Autodesk Inventor part; units mm, degrees
ref_plane "YZ Plane" through (0, 0, 0) normal (1, 0, 0) x (0, 1, 0)
ref_plane "XZ Plane" through (0, 0, 0) normal (0, 1, 0) x (-1, 0, 0)
ref_plane "XY Plane" through (0, 0, 0) normal (0, 0, 1) x (1, 0, 0)
sketch "Sketch1" plane through (0, 0, 0) normal (0, 0, 1) x (1, 0, 0)
  line L0 (0, 0) -> (12, 0)
  line L1 (12, 0) -> (12, 10.5)
  line L2 (12, 10.5) -> (0, 10.5)
  line L3 (0, 10.5) -> (0, 0)
  dimension "d0" = 12
  dimension "d2" = 10.5
extrude "Extrusion1" add sketch "Sketch1" along normal blind 16
fillet "Fillet1" radius 2 4 edges at (12, 10.5, 8) (0, 10.5, 8) (12, 0, 8) (0, 0, 8)
sketch "Sketch2" plane through (0, 0, 16) normal (0, 0, 1) x (1, 0, 0)
  line L0 (12, 2) -> (12, 8.5)
  line L1 (10, 10.5) -> (2, 10.5)
  line L2 (0, 8.5) -> (0, 2)
  line L3 (2, 0) -> (10, 0)
  arc A0 (12, 8.5) -> (10, 10.5) centre (10, 8.5) ccw
  line L4 (12, 8.5) -> (12, 10.5)
  line L5 (12, 10.5) -> (10, 10.5)
  line L6 (2, 10.5) -> (0, 10.5)
  line L7 (0, 10.5) -> (0, 8.5)
  arc A1 (0, 2) -> (2, 0) centre (2, 2) ccw
  line L8 (2, 0) -> (0, 0)
  line L9 (0, 0) -> (2, 0)
  line L10 (12, 2) -> (12, 0)
  arc A2 (10, 0) -> (12, 2) centre (10, 2) ccw
  line L11 (12, 0) -> (10, 0)
  line L12 (0, 0) -> (0, 2)
extrude "Extrusion2" add sketch "Sketch2" along normal blind 9
sketch "Sketch3" plane through (0, 0, 25) normal (0, 0, 1) x (1, 0, 0)
  line L0 (10, 10.5) -> (2, 10.5)
  line L1 (6, 10.5) -> (6, 0)
  line L2 (2, 0) -> (10, 0)
  circle A0 centre (6, 5.25) radius 1.5
  point P0 (0, 0)
  dimension "d8" = 3
extrude "Extrusion3" add sketch "Sketch3" along normal blind 8.5
properties part number "MicroMotor"
Input: part model. Units: mm. Frame: model coordinates. A direction names the side the tool comes from. Coordinates: 2 decimals unless noted, no trailing zeros. Loops run counter-clockwise (first coordinate to the right, second up) from the corner with the lowest first, then second, coordinate; pieces in that order, holes last.
(1) Pull-direction query (Y, two-part tool) for faces 4 (the face through (11.43, 9.9, 8.11)), 5 (the face through (0.4, 0.5, 16)), 6 (the face through (11.4, 0.57, 8.11)); classes: released by +Y, released by -Y, zero draft, split by the parting line, or undercut.
(2) Set-up query: faces 1 (the face through (0.57, 0.6, 8.11)), 2 (the face through (4.6, 6.5, 25)), 3 (the face through (11.5, 10.1, 16)). Return all of +Z, -Z, +X, -X, +Y, -Y with unobstructed straight access to the full face (end or side cutting, diameter ignored); none if empty.
(3) Material intervals for probe 1 along Z at (x, y) = (9, 4.5); probe 2 along Y at (x, z) = (4.75, 31); probe 3 along X at (y, z) = (4.75, 26), sorted ascending.
(4) Section C-C on z = 27. Return the cut outline in (x, y), then the cut area to 3 significant figures.
(5) Section B-B on y = 5.25. Return the cut outline in (x, z).
(6) Section A-A on x = 6. Return the cut outline in (y, z), then the cut area to 3 significant figures.
(7) First-contact query: pin 1 Ø3 at (x, y) = (3.5, 3) entering from +Z; pin 2 Ø1.5 at (y, z) = (1, 5.5) entering from -X. Flat tips, straight axial feed; report the tip coordinate or a pass-through.
(8) Section D-D on x = 3.75. Return the cut outline in (y, z).
Data:
1. face 4: released by +Y
1. face 5: zero draft
1. face 6: released by -Y
2. face 1: -Z, -X, -Y
2. face 2: +Z
2. face 3: -Z, +X, +Y
3. probe 1: z = 0 to 25
3. probe 2: y = 4.42 to 6.08
3. probe 3: x = 4.59 to 7.41
4. outline: circle Ø3 at (6, 5.25)
4. area: 7.07 mm2
5. outline: (0, 0) - (12, 0) - (12, 25) - (7.5, 25) - (7.5, 33.5) - (4.5, 33.5) - (4.5, 25) - (0, 25) - close
6. outline: (0, 0) - (10.5, 0) - (10.5, 25) - (6.75, 25) - (6.75, 33.5) - (3.75, 33.5) - (3.75, 25) - (0, 25) - close
6. area: 288 mm2
7. pin 1: stops at z = 25
7. pin 2: stops at x = 0.02
8. outline: (0, 0) - (10.5, 0) - (10.5, 25) - (0, 25) - close
